Part model, mm, in its own coordinate system. Face numbers are marked on the shaded views. A direction names the side the tool comes from. Give positions to 0.01 mm unless a question says otherwise; leave off trailing zeros. Loops run counter-clockwise (first coordinate to the right, second up) from the corner with the lowest first, then second, coordinate; pieces in that order, holes last. Notation, with made-up numbers: (-27, 1) -> (-18, 1) arc R25 ccw to (-18, 39) -> close; hole circle Ø4 at (48, 8). An arc over 180 degrees is marked (long way). One line per question, with ' | ' between items.
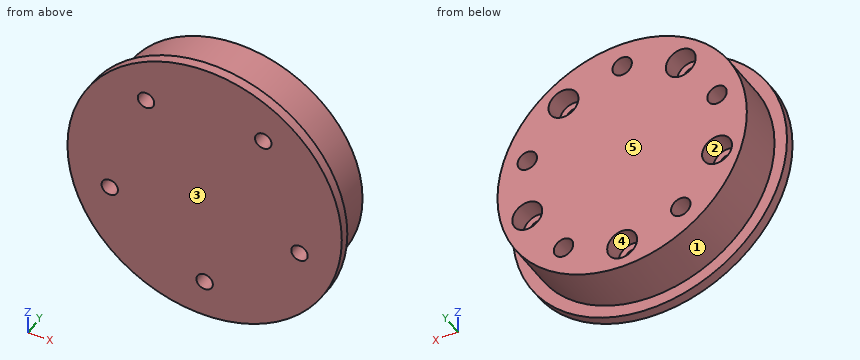
Autodesk Inventor part; units mm, degrees
ref_plane "YZ Plane" through (0, 0, 0) normal (1, 0, 0) x (0, 1, 0)
ref_plane "XZ Plane" through (0, 0, 0) normal (0, 1, 0) x (-1, 0, 0)
ref_plane "XY Plane" through (0, 0, 0) normal (0, 0, 1) x (1, 0, 0)
sketch "Szkic4" plane through (0, 0, 0) normal (0, 1, 0) x (-1, 0, 0)
  circle A0 centre (0, 0) radius 27.5
  dimension "d13" = 55
extrude "Wyciągnięcie proste4" add sketch "Szkic4" along normal blind 2
sketch "Szkic5" plane through (0, 2, 0) normal (0, 1, 0) x (1, 0, 0)
  circle A0 centre (0, 0) radius 25
  dimension "d16" = 50
extrude "Wyciągnięcie proste5" add sketch "Szkic5" along normal blind 10
sketch "Szkic6" plane through (0, 12, 0) normal (0, 1, 0) x (1, 0, 0)
  circle A0 centre (0, 0) radius 20
  circle A1 centre (0, 20) radius 3
  dimension "d19" = 40
  dimension "d20" = 6
extrude "Wyciągnięcie proste6" cut sketch "Szkic6" against normal blind 4 contours A1 A0 | A0 A1 picked at (0, 18.9833) picked at (0.0861, 20.9796)
sketch "Szkic7" plane through (0, 8, -20) normal (0, 1, 0) x (1, 0, 0)
  circle A0 centre (0, 0) radius 1.65
  point P0 (0, -20)
  dimension "d23" = 3.3
extrude "Wyciągnięcie proste7" cut sketch "Szkic7" against normal through all
pattern_circular "Szyk kołowy2" count 5 over 360 about axis through (0, 2, 0) along (0, 1, 0) of "Wyciągnięcie proste6", "Wyciągnięcie proste7"
sketch "Szkic8" plane through (0, 12, 0) normal (0, 1, 0) x (1, 0, 0)
  circle A0 centre (0, 0) radius 20
  circle A1 centre (0, -20) radius 1.95
  dimension "d29" = 40
  dimension "d30" = 3.9
extrude "Wyciągnięcie proste8" cut sketch "Szkic8" against normal blind 8 contours A1 A0 | A0 A1 picked at (0.0759, -19.3474) picked at (0.0638, -20.6398)
pattern_circular "Szyk kołowy3" count 5 over 360 about axis through (0, 2, 0) along (0, 1, 0) of "Wyciągnięcie proste8"
properties part number "_Drukowanie 3D"
1) Pin check, flat tips, straight feed: P1, Ø5, axis at x = -11.76, z = 16.18, coming from the -Y side; P2, Ø2.5, axis at x = -19.02, z = 6.18, coming from the +Y side; P3, Ø5.5, axis at x = 11.76, z = 16.18, coming from the +Y side; P4, Ø2, axis at y = 10, z = -21.5, coming from the -X side. Stop position of each tip, or through.
Found:
P1: y = 0 | P2: y = 4 | P3: y = 8 | P4: x = -14.31
2) Saw through at A-A (x = 0). Give the cut face in (y, z), and give its area (3 significant figures).
Found:
outline: (0, -27.5) -> (2, -27.5) -> (2, -25) -> (12, -25) -> (12, -23) -> (8, -23) -> (8, -21.65) -> (0, -21.65) -> close; (0, -18.35) -> (8, -18.35) -> (8, -17) -> (12, -17) -> (12, 18.05) -> (4, 18.05) -> (4, 21.95) -> (12, 21.95) -> (12, 25) -> (2, 25) -> (2, 27.5) -> (0, 27.5) -> close | area: 528 mm2
3) Drill centre lines: line 1 (Z direction, x = 0, y = 10.75); line 2 (Z direction, x = 19.5, y = 9); line 3 (X direction, y = 7, z = -15). Where is each one in solid material? Low to high.
Found:
line 1: -25 to -23, -17 to 18.05, 21.95 to 25 | line 2: -15.64 to -9.14, -3.22 to 4.29, 8.07 to 15.64 | line 3: -20 to -13.31, -10.2 to 10.2, 13.31 to 20
4) Saw through at C-C (z = 20). Give the cut face in (x, y), and give its area (3 significant figures).
Found:
outline: (-18.87, 0) -> (18.87, 0) -> (18.87, 2) -> (15, 2) -> (15, 12) -> (1.95, 12) -> (1.95, 4) -> (-1.95, 4) -> (-1.95, 12) -> (-15, 12) -> (-15, 2) -> (-18.87, 2) -> close | area: 344 mm2
5) Tool access for the marked faces 4 and 5: list every direction of +Z, -Z, +X, -X, +Y, -Y with a clear straight run to the whole face (end or side of a thin tool).
Found:
face 4: +Y | face 5: +Z, -Z, +X, -X, +Y
6) Pull direction Z, two halves, no side cores. Call the marked faces 1, 2 and 3: pulls with the +Z half, pulls with the -Z half, needs draft (parallel to the pull), parting line crosses it, or undercut.
Found:
face 1: parting line crosses it | face 2: undercut | face 3: needs draft
